Verification items for the finished model (mm, model axes). A direction names the side the tool comes from. Give positions to 0.01 mm unless a question says otherwise; leave off trailing zeros. Order: outer loops, then holes, each group sorted by start corner. A loop starts at its lowest first (then second) coordinate and runs counter-clockwise, first axis right, second up. Notation, with made-up numbers: (-37, 33.5) - (-20, 33.5) arc R34 ccw to (-20, 69.5) - close; hole circle Ø1 at (70.5, 50.25). An arc over 180 degrees is marked (long way). Answer as a JSON object with one key per item and string values.
```python
from build123d import *

# Parameters (mm, degrees)
SKETCH1_R           = 50
SKETCH1_R_2         = 10
BOSS_EXTRUDE2_DEPTH = 10
SKETCH3_R           = 5
CUT_EXTRUDE2_DEPTH  = 10
CIRPATTERN1_COUNT   = 3
SKETCH4_R           = 8
SKETCH4_R_2         = 5
BOSS_EXTRUDE3_DEPTH = 5
CIRPATTERN2_COUNT   = 3


with BuildPart() as part:
    # Sketch1 → Boss-Extrude2 (new body)
    with BuildSketch(Plane.XY):
        Circle(SKETCH1_R)
        Circle(SKETCH1_R_2, mode=Mode.SUBTRACT)
    extrude(amount=BOSS_EXTRUDE2_DEPTH)

    # Sketch3 → Cut-Extrude2 (cut)
    with BuildSketch(Plane.XY):
        with Locations((0, 40)):
            Circle(SKETCH3_R)
    cut_extrude2 = extrude(amount=CUT_EXTRUDE2_DEPTH, mode=Mode.SUBTRACT)

    # CirPattern1: Cut-Extrude2 ×3 about axis
    cirpattern1_axis = Axis((0, 0, 0), (0, 0, 1))
    for i in range(1, CIRPATTERN1_COUNT):
        add(cut_extrude2.rotate(cirpattern1_axis, i * 360 / CIRPATTERN1_COUNT), mode=Mode.SUBTRACT)

    # Sketch4 → Boss-Extrude3 (add)
    with BuildSketch(Plane.XY.offset(10)):
        with Locations((0, 40)):
            Circle(SKETCH4_R)
        with Locations((0, 40)):
            Circle(SKETCH4_R_2, mode=Mode.SUBTRACT)
    boss_extrude3 = extrude(amount=BOSS_EXTRUDE3_DEPTH)

    # CirPattern2: Boss-Extrude3 ×3 about axis
    cirpattern2_axis = Axis((0, 0, 0), (0, 0, 1))
    for i in range(1, CIRPATTERN2_COUNT):
        add(boss_extrude3.rotate(cirpattern2_axis, i * 360 / CIRPATTERN2_COUNT))


solid = part.part
```
(1) Gauge pin test, flat ends, axial feed: pin 1 Ø5 at (y, z) = (-34.5, 4.5) entering from -X; pin 2 Ø5 at (y, z) = (-13, 13.5) entering from -X; pin 3 Ø1 at (x, z) = (30.5, 5) entering from -Y. Record the tip position at first contact, or that the pin passes through.
Computed values:
{"pin 1": "stops at x = -38.42", "pin 2": "stops at x = -41.26", "pin 3": "stops at y = -40"}
(2) Section check D-D (x = -36). Record the cut outline in (y, z).
Computed values:
{"outline": "(-34.7, 0) - (-24.81, 0) - (-24.81, 15) - (-27.88, 15) - (-27.88, 10) - (-34.7, 10) - close; (-15.19, 0) - (34.7, 0) - (34.7, 10) - (-12.12, 10) - (-12.12, 15) - (-15.19, 15) - close"}
(3) Section check C-C (y = -20). Record the cut outline in (x, z).
Computed values:
{"outline": "(-45.83, 0) - (-39.64, 0) - (-39.64, 15) - (-42.64, 15) - (-42.64, 10) - (-45.83, 10) - close; (-29.64, 0) - (29.64, 0) - (29.64, 15) - (26.64, 15) - (26.64, 10) - (-26.64, 10) - (-26.64, 15) - (-29.64, 15) - close; (39.64, 0) - (45.83, 0) - (45.83, 10) - (42.64, 10) - (42.64, 15) - (39.64, 15) - close"}
(4) Section check A-A (y = 40). Record the cut outline in (x, z), then the cut area to 3 significant figures.
Computed values:
{"outline": "(-30, 0) - (-5, 0) - (-5, 15) - (-8, 15) - (-8, 10) - (-30, 10) - close; (5, 0) - (30, 0) - (30, 10) - (8, 10) - (8, 15) - (5, 15) - close", "area": "530 mm²"}
(5) Release check for a two-part mould opening along X. For faces 1 (the cylindrical face through (-27.01, -17.6, 12.46)), 2 (the flat face through (5.2, 40.1, 15)), 3 (the cylindrical face through (47.69, 15.02, 4.93)) record: pulls with the +X half, pulls with the -X half, needs draft (parallel to the pull), parting line crosses it, or undercut.
Computed values:
{"face 1": "undercut", "face 2": "needs draft", "face 3": "parting line crosses it"}
(6) Material ranges on line 1 along Y through (x, z) = (0, 7.25); line 2 along Y through (x, z) = (4, 7); line 3 along Z through (x, y) = (-24, 28.5), recorded low to high. Write a range as [from, to].
Computed values:
{"line 1": "y = [-50, -10], [10, 35], [45, 50]", "line 2": "y = [-49.84, -9.17], [9.17, 37], [43, 49.84]", "line 3": "z = [0, 10]"}
(7) Access from +Z, -Z, +X, -X, +Y, -Y to the whole of each face (thin tool, end or side, straight path). Record for faces 4 (the cylindrical face through (-1.041, 47.932, 12.465)), 5 (the flat face through (33, -15, 15)).
Computed values:
{"face 4": "+Z", "face 5": "+Z, +X, -X, +Y, -Y"}
(8) Section check B-B (x = 0). Record the cut outline in (y, z), then the cut area to 3 significant figures.
Computed values:
{"outline": "(-50, 0) - (-10, 0) - (-10, 10) - (-50, 10) - close; (10, 0) - (35, 0) - (35, 15) - (32, 15) - (32, 10) - (10, 10) - close; (45, 0) - (50, 0) - (50, 10) - (48, 10) - (48, 15) - (45, 15) - close", "area": "730 mm²"}
